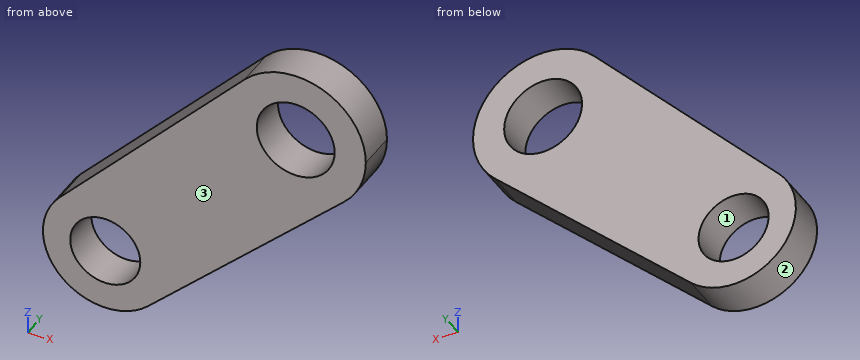
```python
from build123d import *

# Parameters (mm, degrees)
F0_R     = 25
F0_R_2   = 22.5
F1_DEPTH = 25


with BuildPart() as f1:
    # F0 (on Front) → F1 (new body)
    with BuildSketch(Plane.XZ):
        with BuildLine():
            ThreePointArc((30.886308, -32.726686), (41.321204, -17.820159), (45, 0))
            ThreePointArc((45, 0), (16.617748, 41.819259), (-32.726686, 30.886308))
            ThreePointArc((-32.726686, 30.886308), (-31.819805, -31.819805), (30.886308, -32.726686))
        make_face()
        Circle(F0_R, mode=Mode.SUBTRACT)
        with BuildLine():
            ThreePointArc((30.886308, -32.726686), (-31.819805, -31.819805), (-32.726686, 30.886308))
            Line((-32.726686, 30.886308), (-151.347864, -94.80298))
            ThreePointArc((-151.347864, -94.80298), (-107.486144, -85.084801), (-82.257476, -122.257476))
            ThreePointArc((-82.257476, -122.257476), (-85.527517, -138.097618), (-94.80298, -151.347864))
            Line((-94.80298, -151.347864), (30.886308, -32.726686))
        make_face()
        with BuildLine():
            ThreePointArc((-82.257476, -122.257476), (-107.486144, -85.084801), (-151.347864, -94.80298))
            ThreePointArc((-151.347864, -94.80298), (-150.541748, -150.541748), (-94.80298, -151.347864))
            ThreePointArc((-94.80298, -151.347864), (-85.527517, -138.097618), (-82.257476, -122.257476))
        make_face()
        with Locations((-122.257476, -122.257476)):
            Circle(F0_R_2, mode=Mode.SUBTRACT)
    extrude(amount=F1_DEPTH)


solid = f1.part
```
Geometry: final body of the model. Coordinates: model frame, mm. Face numbers are marked on the shaded views. Round coordinates to 2 decimals unless told otherwise and drop trailing zeros. Write each loop counter-clockwise with the first axis right and the second up, starting at its lowest first coordinate (ties: lowest second). Pieces come first, ordered by that corner, then holes.
Item 1: Material intervals for L1, parallel to Z at x = -22, y = -19; L2, parallel to Z at x = 0, y = -17; L3, parallel to X at y = -9.5, z = -9, sorted ascending.
Item 2: Section query B-B (x = 13). Return loops of the section in (y, z), plus the area to 3 significant figures.
Item 3: Section query C-C (y = -8.75). Return loops of the section in (x, z).
Item 4: Pin query (flat end, axial travel): P1, Ø1, axis at x = 1.5, y = -10.5, coming from the -Z side; P2, Ø1.5, axis at x = -36.5, z = -83, coming from the +Y side; P3, Ø3, axis at x = -106, y = -21.5, coming from the +Z side; P4, Ø6, axis at x = -131.5, y = -18, coming from the -Z side. Return the tip coordinate at first contact, or that it passes through.
Item 5: Section query A-A (z = -129.5). Return loops of the section in (x, y) (3 decimals), plus the area to 3 significant figures.
Item 6: Mould query, pull axis Z, two halves, no side actions, for the marked faces 1, 2 and 3. Classes: +Z half, -Z half, draft (parallel to the pull), parting line (faces both ways), or undercut.
Item 7: Section query D-D (z = -83). Return loops of the section in (x, y), plus the area to 3 significant figures.
Completed:
1. L1: z = -82.64 to -11.87, 11.87 to 39.26
1. L2: z = -61.88 to -25, 25 to 45
1. L3: x = -70.37 to -23.32, 23.32 to 44.09
2. outline: (-25, -49.61) - (0, -49.61) - (0, -21.35) - (-25, -21.35) - close; (-25, 21.35) - (0, 21.35) - (0, 43.08) - (-25, 43.08) - close
2. area: 1,250 mm2
3. outline: (-151.35, -94.8) arc R40 ccw to (-94.8, -151.35) - (30.89, -32.73) arc R45 ccw to (45, 0) arc R45 ccw to (-32.73, 30.89) - close; hole circle Ø45 at (-122.26, -122.26); hole circle Ø50 at (0, 0)
4. P1: stops at z = -60.93
4. P2: stops at y = 0
4. P3: stops at z = -45.16
4. P4: stops at z = -161.77
5. outline: (-161.596, -25) - (-143.56, -25) - (-143.56, 0) - (-161.596, 0) - close; (-100.955, -25) - (-71.653, -25) - (-71.653, 0) - (-100.955, 0) - close
5. area: 1,180 mm2
6. face 1: undercut
6. face 2: parting line
6. face 3: draft
7. outline: (-140.21, -25) - (-22.38, -25) - (-22.38, 0) - (-140.21, 0) - close
7. area: 2,950 mm2
